```python
from build123d import *

# Parameters (mm, degrees)
SKETCH1_R             = 100
BOSS_EXTRUDE1_DEPTH   = 14
SKETCH2_R             = 12.5
CUT_EXTRUDE1_DEPTH    = 143.112631388
SKETCH3_R             = 10
CUT_EXTRUDE2_DEPTH    = 11.015412
CIRPATTERN1_START     = 2.984587641
CIRPATTERN1_OUTLINE_R = 10
CIRPATTERN1_DEPTH     = 11.015412359


# Read off the part's stored shape, not the designer's step: CirPattern1
with BuildPart() as part:
    # Sketch1 → Boss-Extrude1 (new body)
    with BuildSketch(Plane(origin=(0, 0, 0), x_dir=(1, 0, 0), z_dir=(0, 1, 0))):
        with Locations(Location((0, 0, 0), (0, 0, 270))):
            Circle(SKETCH1_R)
    extrude(amount=BOSS_EXTRUDE1_DEPTH)

    # Sketch2 → Cut-Extrude1 (cut, through all)
    with BuildSketch(Plane(origin=(0, 0, 0), x_dir=(1, 0, 0), z_dir=(0, 1, 0))):
        with Locations(Location((0, 0, 0), (0, 0, 270))):
            Circle(SKETCH2_R)
    extrude(amount=CUT_EXTRUDE1_DEPTH, mode=Mode.SUBTRACT)

    # Sketch3 → Cut-Extrude2 (cut)
    with BuildSketch(Plane(origin=(0, 14, 0), x_dir=(1, 0, 0), z_dir=(0, 1, 0))):
        with Locations(Location((-23.616715223, 0, 0), (0, 0, 270))):
            Circle(SKETCH3_R)
    extrude(amount=-CUT_EXTRUDE2_DEPTH, mode=Mode.SUBTRACT)

    # CirPattern1 outline → CirPattern1 (cut)
    with BuildSketch(Plane(origin=(0, 0, 0), x_dir=(1, 0, 0), z_dir=(0, 1, 0)).offset(CIRPATTERN1_START)):
        with Locations((0, 23.616715223)):
            Circle(CIRPATTERN1_OUTLINE_R)
        with Locations((23.616715223, 0)):
            Circle(CIRPATTERN1_OUTLINE_R)
        with Locations((0, -23.616715223)):
            Circle(CIRPATTERN1_OUTLINE_R)
    extrude(amount=CIRPATTERN1_DEPTH, mode=Mode.SUBTRACT)


solid = part.part
```
Geometry check sheet. Reference: the model listing, model coordinates, mm. A direction names the side the tool comes from. Coordinates: 2 decimals unless noted, no trailing zeros. Order: outer loops, then holes, each group sorted by start corner. A loop starts at its lowest first (then second) coordinate and runs counter-clockwise, first axis right, second up. Notation, with made-up numbers: (79, 67) - (111, 67) arc R9 ccw to (111, 75) - close; hole circle Ø4 at (84.25, 4). An arc over 180 degrees is marked (long way). Answer as a JSON object with one key per item and string values. Group by question number.
Item 1: Depth check by flat-ended pin: pin 1 Ø20 at (x, z) = (0, 0) entering from +Y; pin 2 Ø1 at (x, y) = (-17, 6) entering from -Z; pin 3 Ø16 at (x, z) = (0, 23.62) entering from -Y; pin 4 Ø8 at (x, y) = (71, 6.5) entering from +Z. Enter the tip coordinate at first touch or a pass-through.
Item 2: Scan lines: probe 1 along X at (y, z) = (11, 0); probe 2 along Z at (x, y) = (-8.5, 5); probe 3 along Z at (x, y) = (-4.5, 13.5). Record each from-to range of solid material in increasing order.
Item 3: Draft check along Z on faces 3 (the face through (-21, 0, -1)), 4 (the face through (33.155, 8.415, -3.004)), 5 (the face through (30.04, 6.9, 95.38)). Enter one of: +Z half, -Z half, draft (parallel to the pull), parting line (faces both ways), or undercut.
Item 4: Sectioned sample at D-D, the plane x = 21.5. Record the cut outline in (y, z), and give its area (3 significant figures).
Item 5: Tool access check on faces 1 (the face through (-21, 14, 21)), 2 (the face through (-7.936, 8.415, -17.532)). Record the directions out of +Z, -Z, +X, -X, +Y, -Y that give a thin tool (end or side, any length) a straight path to the whole face; none if there is none.
Item 6: Sectioned sample at B-B, the plane z = 0. Record the cut outline in (x, y).
Item 7: Sectioned sample at C-C, the plane y = 10.75. Record the cut outline in (x, z), and give its area (3 significant figures).
Item 8: Sectioned sample at A-A, the plane x = 0. Record the cut outline in (y, z).
Resolved:
{
 "1": {"pin 1": "through", "pin 2": "z = -98.63", "pin 3": "y = 0", "pin 4": "z = 74.24"},
 "2": {"probe 1": "-100 to -33.62, -13.62 to -12.5, 12.5 to 13.62, 33.62 to 100", "probe 2": "-99.64 to -28.88, -18.35 to -9.17, 9.17 to 18.35, 28.88 to 99.64", "probe 3": "-99.9 to -32.55, -14.69 to -11.66, 11.66 to 14.69, 32.55 to 99.9"},
 "3": {"face 3": "draft", "face 4": "undercut", "face 5": "parting line"},
 "4": {"outline": "(0, -97.66) - (14, -97.66) - (14, -9.77) - (2.98, -9.77) - (2.98, 9.77) - (14, 9.77) - (14, 97.66) - (0, 97.66) - close", "area": "2,520 mm^2"},
 "5": {"face 1": "+Z, -Z, +X, -X, +Y", "face 2": "+Y"},
 "6": {"outline": "(-100, 0) - (-12.5, 0) - (-12.5, 14) - (-13.62, 14) - (-13.62, 2.98) - (-33.62, 2.98) - (-33.62, 14) - (-100, 14) - close; (12.5, 0) - (100, 0) - (100, 14) - (33.62, 14) - (33.62, 2.98) - (13.62, 2.98) - (13.62, 14) - (12.5, 14) - close"},
 "7": {"outline": "circle Ø200 at (0, 0); hole circle Ø20 at (-23.62, 0); hole circle Ø25 at (0, 0); hole circle Ø20 at (0, -23.62); hole circle Ø20 at (0, 23.62); hole circle Ø20 at (23.62, 0)", "area": "29,700 mm^2"},
 "8": {"outline": "(0, -100) - (14, -100) - (14, -33.62) - (2.98, -33.62) - (2.98, -13.62) - (14, -13.62) - (14, -12.5) - (0, -12.5) - close; (0, 12.5) - (14, 12.5) - (14, 13.62) - (2.98, 13.62) - (2.98, 33.62) - (14, 33.62) - (14, 100) - (0, 100) - close"}
}
